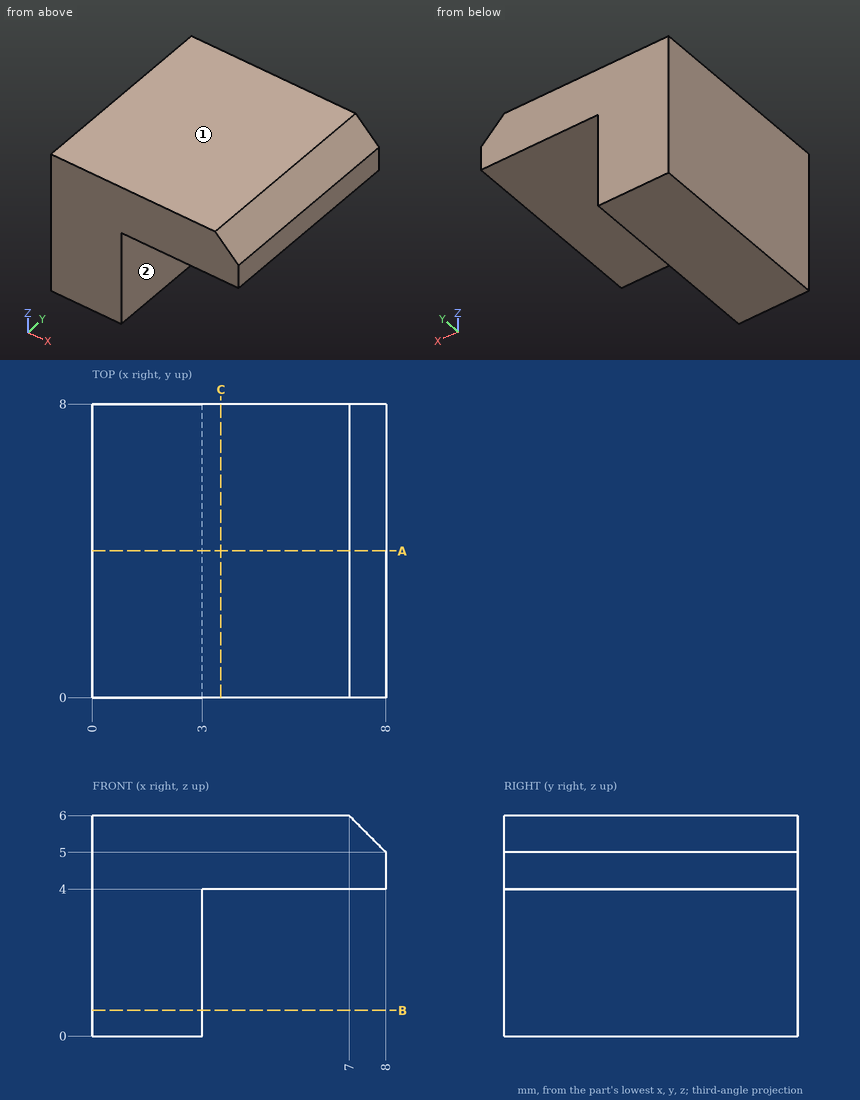
Study the drawing (mm; zero at the part's minimum x, y, z) and answer. A direction names the side the tool comes from. Give positions to 0.01 mm unless a question says otherwise; leave off trailing zeros. Loops run counter-clockwise (first coordinate to the right, second up) from the corner with the lowest first, then second, coordinate; pieces in that order, holes last. Notation, with made-up numbers: (-1, 84.5) - (53, 84.5) arc R30 cw to (53, 111.5) - close; hole circle Ø8 at (-6.75, 60). An arc over 180 degrees is marked (long way). Answer as CSV lines item,"result". Start each with the question number.
1) Which of the six approach directions +Z, -Z, +X, -X, +Y, -Y give full straight-line access (tool end or side, diameter ignored) to the marked faces 1 and 2?
2) Each of these flat-tipped pins is pushed along its axis until it touches: pin 1 Ø4 at (x, y) = (5.5, 2.5) entering from -Z; pin 2 Ø1.2 at (y, z) = (5.5, 1.5) entering from +X. Where does it stop, or does it pass through?
3) Find section A-A (y = 4). Write down the section's boundary in (x, z), then the cut area to 3 significant figures.
4) Find section C-C (x = 3.5). Write down the section's boundary in (y, z).
5) Find section B-B (z = 0.7). Write down the section's boundary in (x, y).
6) Straight lines are drawn through the part: L1, parallel to Z at x = 5.5, y = 4; L2, parallel to X at y = 4.5, z = 3.5; L3, parallel to X at y = 1, z = 5.1. For each, find the intervals that lie inside material, in ascending order. Write a range as from..to.
Findings below:
1,face 1,"+Z, +X, -X, +Y, -Y"
1,face 2,"-Z, +X, +Y, -Y"
2,pin 1,"z = 4"
2,pin 2,"x = 3"
3,outline,"(0, 0) - (3, 0) - (3, 4) - (8, 4) - (8, 5) - (7, 6) - (0, 6) - close"
3,area,"27.5 mm^2"
4,outline,"(0, 4) - (8, 4) - (8, 6) - (0, 6) - close"
5,outline,"(0, 0) - (3, 0) - (3, 8) - (0, 8) - close"
6,L1,"4..6"
6,L2,"0..3"
6,L3,"0..7.9"
